Source: CAD feature listing. Evaluate the final solid. Frame: model axes, mm. A direction names the side the tool comes from. Round coordinates to 2 decimals unless told otherwise and drop trailing zeros. Order: outer loops, then holes, each group sorted by start corner. A loop starts at its lowest first (then second) coordinate and runs counter-clockwise, first axis right, second up. Notation, with made-up numbers: (32, -21) - (82, -21) arc R36 cw to (82, 13) - close; hole circle Ø2 at (5.5, 40). An arc over 180 degrees is marked (long way). Return JSON: item names as keys, results as strings. Group by question number.
1) Section A-A, the plane z = -31.5. Return loops of the section in (x, y), plus the area to 3 significant figures.
2) Contact query for flat-ended pins moving along their axis: P1, Ø3, axis at x = 0, y = 52, coming from the +Z side; P2, Ø1.5, axis at y = 116, z = 30, coming from the +X side; P3, Ø12, axis at y = 102.5, z = -40, coming from the -X side. Output: stop coordinate, or through.
3) Access query for faces 4 (the flat face through (5.55, 1.25, 30.37)), 5 (the flat face through (38, 0, 6)), 6 (the flat face through (-5.55, 186.71, -30.37)). Directions: +Z, -Z, +X, -X, +Y, -Y. A direction counts if a zero-diameter tool reaches every point of the face in a straight line with its end or side. Return the directions, or none.
4) Section B-B, the plane y = 170.5. Return loops of the section in (x, z).
5) Section D-D, the plane z = -48. Return loops of the section in (x, y), plus the area to 3 significant figures.
6) Ray query, line 1 (Y direction, x = -33, z = 38); line 2 (X direction, y = 145, z = -11.5); line 3 (X direction, y = 83.5, z = 47). Return the intervals inside material, ascending. Write a range as from..to.
7) Section C-C, the plane x = -30.5. Return loops of the section in (y, z).
8) Mould query, pull axis X, two halves, no side actions, for faces 1 (the flat face through (38, 187.96, 6)), 2 (the cylindrical face through (-13.49, 92.66, 60.75)), 3 (the flat face through (-1, 185.42, 1)). Classes: pulls with the +X half, pulls with the -X half, needs draft (parallel to the pull), parting line crosses it, or undercut.
```python
from build123d import *

# Parameters (mm, degrees)
SKETCH1_R            = 62.23
BOSS_EXTRUDE1_DEPTH  = 187.96
CUT_EXTRUDE7_DEPTH   = 2.54
CIRPATTERN2_COUNT    = 4
MIRROR1_COPY_1_DEPTH = 2.54
MIRROR1_COPY_2_DEPTH = 2.54
MIRROR1_COPY_3_DEPTH = 2.54


with BuildPart() as part:
    # Sketch1 → Boss-Extrude1 (new body)
    with BuildSketch(Plane(origin=(0, 0, 0), x_dir=(1, 0, 0), z_dir=(0, 1, 0))):
        Circle(SKETCH1_R)
    extrude(amount=BOSS_EXTRUDE1_DEPTH)

    # Sketch2 → Cut-Extrude7 (cut)
    with BuildSketch(Plane(origin=(0, 187.96, 0), x_dir=(1, 0, 0), z_dir=(0, 1, 0))):
        with BuildLine():
            Line((-34.977816307, -51.46965384), (0.021593035, -0.253080503))
            ThreePointArc((0.021593035, -0.253080503), (-0.212652586, -0.138906004), (-0.223069042, 0.12147511))
            Line((-0.223069042, 0.12147511), (-61.186975042, -11.345791522))
            ThreePointArc((-61.186975042, -11.345791522), (-52.099883451, -34.031970915), (-34.977816307, -51.46965384))
        make_face()
    cut_extrude7 = extrude(amount=-CUT_EXTRUDE7_DEPTH, mode=Mode.SUBTRACT)

    # CirPattern2: Cut-Extrude7 ×4 about axis
    cirpattern2_axis = Axis((0, 0, 0), (0, 1, 0))
    for i in range(1, CIRPATTERN2_COUNT):
        add(cut_extrude7.rotate(cirpattern2_axis, i * 360 / CIRPATTERN2_COUNT), mode=Mode.SUBTRACT)

    # Mirror1: Cut-Extrude7 across plane
    add(cut_extrude7.mirror(Plane.ZX.offset(93.98)), mode=Mode.SUBTRACT)

    # Mirror1 copy 1 sketch → Mirror1 copy 1 (cut)
    with BuildSketch(Plane(origin=(0, 0, 0), x_dir=(0, 0, -1), z_dir=(0, -1, 0))):
        with BuildLine():
            Line((-34.977816307, 51.46965384), (0.021593035, 0.253080503))
            ThreePointArc((0.021593035, 0.253080503), (-0.212652586, 0.138906004), (-0.223069042, -0.12147511))
            Line((-0.223069042, -0.12147511), (-61.186975042, 11.345791522))
            ThreePointArc((-61.186975042, 11.345791522), (-52.099883451, 34.031970915), (-34.977816307, 51.46965384))
        make_face()
    extrude(amount=-MIRROR1_COPY_1_DEPTH, mode=Mode.SUBTRACT)

    # Mirror1 copy 2 sketch → Mirror1 copy 2 (cut)
    with BuildSketch(Plane(origin=(0, 0, 0), x_dir=(-1, 0, 0), z_dir=(0, -1, 0))):
        with BuildLine():
            Line((-34.977816307, 51.46965384), (0.021593035, 0.253080503))
            ThreePointArc((0.021593035, 0.253080503), (-0.212652586, 0.138906004), (-0.223069042, -0.12147511))
            Line((-0.223069042, -0.12147511), (-61.186975042, 11.345791522))
            ThreePointArc((-61.186975042, 11.345791522), (-52.099883451, 34.031970915), (-34.977816307, 51.46965384))
        make_face()
    extrude(amount=-MIRROR1_COPY_2_DEPTH, mode=Mode.SUBTRACT)

    # Mirror1 copy 3 sketch → Mirror1 copy 3 (cut)
    with BuildSketch(Plane(origin=(0, 0, 0), x_dir=(0, 0, 1), z_dir=(0, -1, 0))):
        with BuildLine():
            Line((-34.977816307, 51.46965384), (0.021593035, 0.253080503))
            ThreePointArc((0.021593035, 0.253080503), (-0.212652586, 0.138906004), (-0.223069042, -0.12147511))
            Line((-0.223069042, -0.12147511), (-61.186975042, 11.345791522))
            ThreePointArc((-61.186975042, 11.345791522), (-52.099883451, 34.031970915), (-34.977816307, 51.46965384))
        make_face()
    extrude(amount=-MIRROR1_COPY_3_DEPTH, mode=Mode.SUBTRACT)


solid = part.part
```
Geometry check:
{
 "1": {"outline": "(-53.67, 0) - (-46.38, 0) - (-46.38, 2.54) - (-5.76, 2.54) - (-5.76, 0) - (21.33, 0) - (21.33, 2.54) - (53.67, 2.54) - (53.67, 185.42) - (21.33, 185.42) - (21.33, 187.96) - (-5.76, 187.96) - (-5.76, 185.42) - (-46.38, 185.42) - (-46.38, 187.96) - (-53.67, 187.96) - close", "area": "19,800 mm2"},
 "2": {"P1": "z = 62.23", "P2": "x = 54.93", "P3": "x = -52.12"},
 "3": {"face 4": "-Y", "face 5": "+Z, -Z, +X, -X, -Y", "face 6": "+Y"},
 "4": {"outline": "circle Ø124.46 at (0, 0)"},
 "5": {"outline": "(-39.61, 2.54) - (-8.87, 2.54) - (-8.87, 0) - (32.61, 0) - (32.61, 2.54) - (39.61, 2.54) - (39.61, 185.42) - (32.61, 185.42) - (32.61, 187.96) - (-8.87, 187.96) - (-8.87, 185.42) - (-39.61, 185.42) - close", "area": "14,700 mm2"},
 "6": {"line 1": "2.54..185.42", "line 2": "-61.16..61.16", "line 3": "-40.79..40.79"},
 "7": {"outline": "(0, -20.65) - (2.54, -20.65) - (2.54, -54.24) - (185.42, -54.24) - (185.42, -20.65) - (187.96, -20.65) - (187.96, 5.57) - (185.42, 5.57) - (185.42, 44.92) - (187.96, 44.92) - (187.96, 54.24) - (0, 54.24) - (0, 44.92) - (2.54, 44.92) - (2.54, 5.57) - (0, 5.57) - close"},
 "8": {"face 1": "needs draft", "face 2": "parting line crosses it", "face 3": "undercut"}
}
